CAD build for the part. Positions are in the model's coordinates, mm. A direction names the side the tool comes from. Coordinates: 2 decimals unless noted, no trailing zeros. Loops run counter-clockwise (first coordinate to the right, second up) from the corner with the lowest first, then second, coordinate; pieces in that order, holes last.
1) Saw through at A-A, the plane z = 1.7. Write the cut outline in (x, y).
2) Pin check, flat tips, straight feed: pin 1 Ø1 at (x, z) = (35.5, 1.5) entering from -Y; pin 2 Ø1 at (y, z) = (4.5, 2) entering from -X; pin 3 Ø1 at (x, z) = (22, 2) entering from -Y. Stop position of each tip, or through.
3) Which spindle directions (+Z, -Z, +X, -X, +Y, -Y) get a long thin tool onto all of the face, cutting with end or side? Do faces 1 (the cylindrical face through (163.36, 54.14, 1.63)), 2 (the flat face through (21, 9.766, 2)), 3 (the flat face through (159.525, 5, 2)). Say none if no direction does.
4) Two-plate mould, pull along Y, no slides. Class faces 4 (the flat face through (92, 60.566, 2)), 5 (the cylindrical face through (21.05, 17.74, 1.63)), 6 (the flat face through (170.493, 34, 2)): +Y half, -Y half, draft (parallel to the pull), parting line (faces both ways), or undercut.
5) Wall check: line 1 along X through (y, z) = (54, 2.05); line 2 along Y through (x, z) = (162, 2.3); line 3 along X through (y, z) = (17.5, 2.9). Give the ranges that are in metal, low to high.
Autodesk Inventor part; units mm, degrees
ref_plane "YZ Plane" through (0, 0, 0) normal (1, 0, 0) x (0, 1, 0)
ref_plane "XZ Plane" through (0, 0, 0) normal (0, 1, 0) x (-1, 0, 0)
ref_plane "XY Plane" through (0, 0, 0) normal (0, 0, 1) x (1, 0, 0)
sketch "Sketch1" plane through (0, 0, 0) normal (0, 0, 1) x (1, 0, 0)
  line L0 (15.0622, 60.5663) -> (170.4927, 60.5663)
  line L1 (170.4927, 60.5663) -> (170.4927, 9.7663)
  line L2 (15.0622, 9.7663) -> (15.0622, 60.5663)
  line L3 (170.4927, 9.7663) -> (170.4927, 6.5913)
  line L4 (26.4922, 6.5913) -> (26.4922, 9.7663)
  line L5 (159.5247, 6.5913) -> (159.5247, 3.4163)
  line L6 (159.5247, 3.4163) -> (42.0497, 3.4163)
  line L7 (42.0497, 3.4163) -> (42.0497, 6.5913)
  circle A0 centre (21.4122, 54.2163) radius 1.651
  circle A1 centre (21.4122, 16.129) radius 1.651
  circle A2 centre (165.0087, 16.129) radius 1.651
  circle A3 centre (165.0087, 54.2163) radius 1.651
  line L8 (33.3756, 50.5714) -> (117.4496, 50.5714)
  line L9 (117.4496, 50.5714) -> (117.4496, 28.8544)
  line L10 (117.4496, 28.8544) -> (33.3756, 28.8544)
  line L11 (33.3756, 28.8544) -> (33.3756, 50.5714)
  line L12 (39.2811, 23.114) -> (50.0761, 23.114)
  line L13 (50.0761, 23.114) -> (50.0761, 12.319)
  line L14 (50.0761, 12.319) -> (39.2811, 12.319)
  line L15 (39.2811, 12.319) -> (39.2811, 23.114)
  line L16 (54.6481, 23.114) -> (65.4431, 23.114)
  line L17 (65.4431, 23.114) -> (65.4431, 12.319)
  line L18 (65.4431, 12.319) -> (54.6481, 12.319)
  line L19 (54.6481, 12.319) -> (54.6481, 23.114)
  line L20 (70.0151, 23.114) -> (80.8101, 23.114)
  line L21 (80.8101, 23.114) -> (80.8101, 12.319)
  line L22 (80.8101, 12.319) -> (70.0151, 12.319)
  line L23 (70.0151, 12.319) -> (70.0151, 23.114)
  line L24 (85.3821, 23.114) -> (96.1771, 23.114)
  line L25 (96.1771, 23.114) -> (96.1771, 12.319)
  line L26 (96.1771, 12.319) -> (85.3821, 12.319)
  line L27 (85.3821, 12.319) -> (85.3821, 23.114)
  line L28 (100.7491, 23.114) -> (111.5441, 23.114)
  line L29 (111.5441, 23.114) -> (111.5441, 12.319)
  line L30 (111.5441, 12.319) -> (100.7491, 12.319)
  line L31 (100.7491, 12.319) -> (100.7491, 23.114)
  line L32 (138.7221, 23.114) -> (149.5171, 23.114)
  line L33 (149.5171, 23.114) -> (149.5171, 12.319)
  line L34 (149.5171, 12.319) -> (138.7221, 12.319)
  line L35 (138.7221, 12.319) -> (138.7221, 23.114)
  line L36 (170.4927, 9.7663) -> (170.4927, 9.7663)
  line L37 (26.4922, 9.7663) -> (15.0622, 9.7663)
  line L38 (26.4922, 6.5913) -> (42.0497, 6.5913)
  line L39 (159.5247, 6.5913) -> (170.4927, 6.5913)
  circle A4 centre (144.1196, 41.5163) radius 3.4925
  line L40 (144.1196, 23.114) -> (144.1196, 12.319)
  circle A5 centre (44.6786, 17.7165) radius 5.3975
  circle A6 centre (60.0456, 17.7165) radius 5.3975
  circle A7 centre (75.4126, 17.7165) radius 5.3975
  circle A8 centre (90.7796, 17.7165) radius 5.3975
  circle A9 centre (106.1466, 17.7165) radius 5.3975
  circle A10 centre (144.1196, 17.7165) radius 5.3975
  dimension "d0" = 3.302
  dimension "d1" = 6.35
  dimension "d2" = 6.35
  dimension "d3" = 84.074
  dimension "d4" = 21.717
  dimension "d5" = 10.795
  dimension "d6" = 10.795
  dimension "d7" = 10.795
  dimension "d8" = 10.795
  dimension "d9" = 10.795
  dimension "d10" = 10.795
  dimension "d11" = 10.795
  dimension "d12" = 4.572
  dimension "d13" = 4.572
  dimension "d14" = 4.572
  dimension "d15" = 4.572
  dimension "d16" = 5.9055
  dimension "d17" = 5.9055
  dimension "d21" = 6.985
  dimension "d22" = 26.67
  dimension "d25" = 0
  dimension "d26" = 3.302
  dimension "d28" = 3.302
  dimension "d32" = 50.8
  dimension "d33" = 155.4305
  dimension "d34" = 6.35
  dimension "d39" = 26.373
  dimension "d40" = 19.05
  dimension "d41" = 29.6164
  dimension "d43" = 15.367
  dimension "d44" = 37.973
sketch "Sketch2" plane through (0, 0, 0) normal (0, 0, 1) x (1, 0, 0)
  line L0 (15.0622, 9.7663) -> (15.0622, 60.5663)
  line L1 (15.0622, 60.5663) -> (170.4927, 60.5663)
  line L2 (33.3756, 50.5714) -> (117.4496, 50.5714)
  line L3 (117.4496, 50.5714) -> (117.4496, 28.8544)
  line L4 (170.4927, 60.5663) -> (170.4927, 9.7663)
  line L5 (159.5247, 6.5913) -> (170.4927, 6.5913)
  line L6 (159.5247, 6.5913) -> (159.5247, 3.4163)
  line L7 (159.5247, 3.4163) -> (42.0497, 3.4163)
  line L8 (42.0497, 3.4163) -> (42.0497, 6.5913)
  line L9 (26.4922, 6.5913) -> (42.0497, 6.5913)
  line L10 (26.4922, 6.5913) -> (26.4922, 9.7663)
  line L11 (26.4922, 9.7663) -> (15.0622, 9.7663)
  circle A0 centre (21.4122, 16.129) radius 1.651
  circle A1 centre (21.4122, 54.2163) radius 1.651
  circle A2 centre (165.0087, 54.2163) radius 1.651
  circle A3 centre (165.0087, 16.129) radius 1.651
  line L12 (15.0622, 60.5663) -> (15.0622, 9.7663)
  line L13 (15.0622, 9.7663) -> (26.4922, 9.7663)
  line L14 (26.4922, 9.7663) -> (26.4922, 6.5913)
  line L15 (26.4922, 6.5913) -> (42.0497, 6.5913)
  line L16 (42.0497, 6.5913) -> (42.0497, 3.4163)
  line L17 (42.0497, 3.4163) -> (159.5247, 3.4163)
  line L18 (159.5247, 3.4163) -> (159.5247, 6.5913)
  line L19 (159.5247, 6.5913) -> (170.4927, 6.5913)
  line L20 (170.4927, 6.5913) -> (170.4927, 60.5663)
  line L21 (170.4927, 60.5663) -> (15.0622, 60.5663)
  circle A4 centre (21.4122, 54.2163) radius 1.651
  circle A5 centre (21.4122, 16.129) radius 1.651
  circle A6 centre (165.0087, 16.129) radius 1.651
  circle A7 centre (165.0087, 54.2163) radius 1.651
  point P0 (0, 0)
  point P1 (144.1196, 41.5163)
surface extrude "ExtrusionSrf1" sketch "Sketch1" along normal blind 3.302 shown yes curves L0 L1 L36 L3 L39 L5 L6 L7 L38 L4 L37 L2
extrude "Extrusion1" add sketch "Sketch2" along normal blind 3.302
equation "\"d35\" = d28"
equation "\"d37\" = d28"
properties part number "FP_PCB"
Data:
1. outline: (15.06, 9.77) - (26.49, 9.77) - (26.49, 6.59) - (42.05, 6.59) - (42.05, 3.42) - (159.52, 3.42) - (159.52, 6.59) - (170.49, 6.59) - (170.49, 60.57) - (15.06, 60.57) - close; hole circle Ø3.3 at (21.41, 16.13); hole circle Ø3.3 at (21.41, 54.22); hole circle Ø3.3 at (165.01, 16.13); hole circle Ø3.3 at (165.01, 54.22)
2. pin 1: stops at y = 6.59
2. pin 2: stops at x = 42.05
2. pin 3: stops at y = 9.77
3. face 1: +Z, -Z
3. face 2: +Z, -Z, -X, -Y
3. face 3: +Z, -Z, +X, -Y
4. face 4: +Y half
4. face 5: undercut
4. face 6: draft
5. line 1: x = 15.06 to 19.78, 23.05 to 163.37, 166.65 to 170.49
5. line 2: y = 6.59 to 60.57
5. line 3: x = 15.06 to 20.49, 22.33 to 164.09, 165.93 to 170.49
